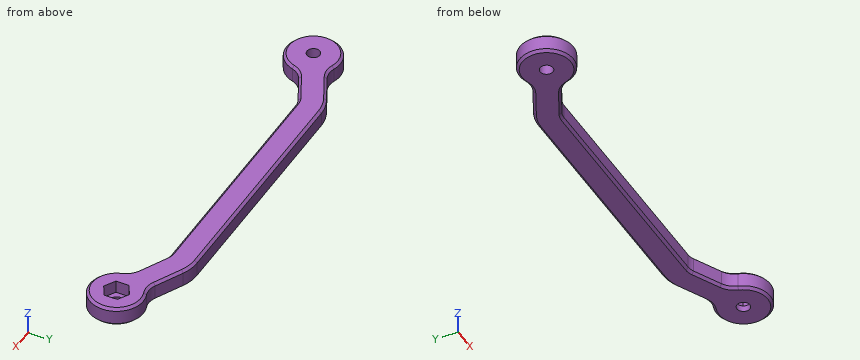
```python
from build123d import *

# Parameters (mm, degrees)
SKETCH1_R           = 2.05
BOSS_EXTRUDE1_DEPTH = 6
CUT_EXTRUDE1_DEPTH  = 4
CHAMFER3_SIZE       = 0.8


with BuildPart() as part:
    # Sketch1 → Boss-Extrude1 (new body)
    with BuildSketch(Plane.XY):
        with BuildLine():
            Line((-52.397368877, 8.273451517), (-43.689164944, 12.627553483))
            ThreePointArc((-43.689164944, 12.627553483), (-40.86217617, 13.652236863), (-37.875388203, 14))
            Line((-37.875388203, 14), (37.875388203, 14))
            ThreePointArc((37.875388203, 14), (40.86217617, 13.652236863), (43.689164944, 12.627553483))
            Line((43.689164944, 12.627553483), (52.397368877, 8.273451517))
            ThreePointArc((52.397368877, 8.273451517), (54.728318318, 7.650368424), (57.116243367, 7.995870664))
            ThreePointArc((57.116243367, 7.995870664), (67.602631123, -3.801315562), (51.873049489, -2.490517092))
            ThreePointArc((51.873049489, -2.490517092), (50.716696252, -0.372875708), (48.819660113, 1.118033989))
            Line((48.819660113, 1.118033989), (40.11145618, 5.472135955))
            ThreePointArc((40.11145618, 5.472135955), (39.024152805, 5.866244947), (37.875388203, 6))
            Line((37.875388203, 6), (-37.875388203, 6))
            ThreePointArc((-37.875388203, 6), (-39.024152805, 5.866244947), (-40.11145618, 5.472135955))
            Line((-40.11145618, 5.472135955), (-48.819660113, 1.118033989))
            ThreePointArc((-48.819660113, 1.118033989), (-50.716696252, -0.372875708), (-51.873049489, -2.490517092))
            ThreePointArc((-51.873049489, -2.490517092), (-67.602631123, -3.801315562), (-57.116243367, 7.995870664))
            ThreePointArc((-57.116243367, 7.995870664), (-54.728318318, 7.650368424), (-52.397368877, 8.273451517))
        make_face()
        with Locations((-60, 0)):
            Circle(SKETCH1_R, mode=Mode.SUBTRACT)
        with Locations((60, 0)):
            Circle(SKETCH1_R, mode=Mode.SUBTRACT)
    extrude(amount=BOSS_EXTRUDE1_DEPTH)

    # Sketch3 → Cut-Extrude1 (cut)
    with BuildSketch(Plane.XY.offset(6)):
        Polygon((60, 4.099186911), (56.45, 2.049593456), (56.45, -2.049593456), (60, -4.099186911), (63.55, -2.049593456), (63.55, 2.049593456), align=None)
    extrude(amount=-CUT_EXTRUDE1_DEPTH, mode=Mode.SUBTRACT)

    # Chamfer3
    chamfer3_edges = [part.edges().sort_by_distance(p)[0] for p in [
        (-40.86217617, 13.652236863, 6),
        (48.04326691, 10.4505025, 0),
        (54.728318318, 7.650368424, 0),
        (67.602631123, -3.801315562, 0),
        (-48.04326691, 10.4505025, 6),
        (50.716696252, -0.372875708, 0),
        (44.465558146, 3.295084972, 0),
        (39.024152805, 5.866244947, 0),
        (0, 6, 0),
        (-39.024152805, 5.866244947, 0),
        (-44.465558146, 3.295084972, 0),
        (-50.716696252, -0.372875708, 0),
        (-67.602631123, -3.801315562, 0),
        (-54.728318318, 7.650368424, 0),
        (-48.04326691, 10.4505025, 0),
        (-54.728318318, 7.650368424, 6),
        (-40.86217617, 13.652236863, 0),
        (0, 14, 0),
        (40.86217617, 13.652236863, 0),
        (-67.602631123, -3.801315562, 6),
        (-50.716696252, -0.372875708, 6),
        (-44.465558146, 3.295084972, 6),
        (-39.024152805, 5.866244947, 6),
        (0, 6, 6),
        (39.024152805, 5.866244947, 6),
        (44.465558146, 3.295084972, 6),
        (40.86217617, 13.652236863, 6),
        (50.716696252, -0.372875708, 6),
        (67.602631123, -3.801315562, 6),
        (54.728318318, 7.650368424, 6),
        (48.04326691, 10.4505025, 6),
        (0, 14, 6),
    ]]
    chamfer(chamfer3_edges, length=CHAMFER3_SIZE)


solid = part.part
```
Here's how the part is built. I have some questions about the finished solid (model axes, mm). Give positions to 0.01 mm unless a question says otherwise; leave off trailing zeros. Order: outer loops, then holes, each group sorted by start corner. A loop starts at its lowest first (then second) coordinate and runs counter-clockwise, first axis right, second up. Notation, with made-up numbers: (63.25, -15.5) -> (77.25, -15.5) arc R11 ccw to (77.25, -0.5) -> close; hole circle Ø4 at (11.25, -27). An arc over 180 degrees is marked (long way). Use CSV: the item, a comma, the result in double quotes. Start each with the question number.
Item 1: Suppose I cut it at B-B (x = 31). List the corners of the cut face in (y, z) for me.
Item 2: Suppose I cut it at D-D (y = 0). Give the number of separate pieces and of enclosed holes in the cut face, and give its area (3 significant figures).
Item 3: Suppose I cut it at C-C (y = 10.75). List the corners of the cut face in (x, z) for me, and give its area (3 significant figures).
Item 4: I'm going to push flat-ended pins straight in: P1, Ø3.5, axis at x = 11.5, z = 3.5, coming from the -Y side; P2, Ø2.5, axis at x = 60, y = 0, coming from the +Z side; P3, Ø1, axis at y = -2.5, z = 1, coming from the -X side; P4, Ø2, axis at y = 11, z = 5, coming from the -X side. Where does each tip first touch, or does it pass through?
Item 5: Suppose I cut it at A-A (x = -60). List the corners of the cut face in (y, z) for me.
Item 6: If I drill on probe 1 along Y at (x, z) = (-60, 1.6); probe 2 along X at (y, z) = (2.5, 5.5); probe 3 along X at (y, z) = (-2.75, 2.25), over which ranges is the centre line in solid material (lowest first)? Write a range as [from, to].
Answer block:
1,outline,"(6, 0.8) -> (6.8, 0) -> (13.2, 0) -> (14, 0.8) -> (14, 5.2) -> (13.2, 6) -> (6.8, 6) -> (6, 5.2) -> close"
2,separate pieces,"4"
2,enclosed holes,"0"
2,area,"153 mm^2"
3,outline,"(-47.44, 0.8) -> (-45.66, 0) -> (45.66, 0) -> (47.44, 0.8) -> (47.44, 5.2) -> (45.66, 6) -> (-45.66, 6) -> (-47.44, 5.2) -> close"
3,area,"566 mm^2"
4,P1,"stops at y = 6"
4,P2,"passes through"
4,P3,"stops at x = -68.26"
4,P4,"stops at x = -48.94"
5,outline,"(-8.5, 0.8) -> (-7.7, 0) -> (-2.05, 0) -> (-2.05, 6) -> (-7.7, 6) -> (-8.5, 5.2) -> close; (2.05, 0) -> (7.7, 0) -> (8.5, 0.8) -> (8.5, 5.2) -> (7.7, 6) -> (2.05, 6) -> close"
6,probe 1,"y = [-8.5, -2.05], [2.05, 8.5]"
6,probe 2,"x = [-67.81, -46.73], [46.73, 57.23], [62.77, 67.81]"
6,probe 3,"x = [-68.04, -51.96], [51.96, 57.66], [62.34, 68.04]"
